Here's how the part is built. I have some questions about the finished solid (model axes, mm). A direction names the side the tool comes from. Coordinates: 2 decimals unless noted, no trailing zeros. Order: outer loops, then holes, each group sorted by start corner. A loop starts at its lowest first (then second) coordinate and runs counter-clockwise, first axis right, second up. Notation, with made-up numbers: (53, 87.5) - (91, 87.5) arc R8 cw to (91, 97.5) - close; hole circle Ø1 at (-25.5, -36). An arc over 180 degrees is marked (long way). Answer in a Markdown table with one row per item. Add a question column.
Item 1: Will these pins go through, and if not, where does the flat tip stop? pin 1 Ø4 at (x, z) = (85, 4) entering from -Y; pin 2 Ø1.5 at (x, z) = (6.5, 4) entering from -Y; pin 3 Ø3.5 at (y, z) = (44.5, 3) entering from -X; pin 4 Ø2.5 at (y, z) = (72.5, 4) entering from -X.
Item 2: I want a section at C-C (y = 18). Please give me the cut outline in (x, z).
Item 3: I want a section at D-D (x = 6). Please give me the cut outline in (y, z), plus the area to 3 significant figures.
Item 4: I want a section at B-B (z = 4). Count the separate pieces of the cut face and the enclosed holes in it, plus the area to 3 significant figures.
Item 5: If I drill on line 1 along Z through (x, y) = (6, 11); line 2 along X through (y, z) = (13.5, 3.5); line 3 along Y through (x, z) = (90, 6.75), over which ranges is the centre line in solid material (lowest first)? Write a range as from..to.
Item 6: I want a section at A-A (x = 20). Please give me the cut outline in (y, z), plus the area to 4 significant figures.
Item 7: On a 3-axis mill with a long thin cutter (end or side, diameter ignored), from which of +Z, -Z, +X, -X, +Y, -Y can I reach the whole of each face in a straight line? I mean faces 5 (the flat face through (85, 45, 4)), 6 (the flat face through (26, 52, 4)), 7 (the cylindrical face through (80.942, 14.35, 2.465)), 8 (the cylindrical face through (56, 37.8, 3.9)). Say none if no direction works.
Item 8: Thinking about a two-plate mould opening in X: for faces 1 (the cylindrical face through (56, 49.2, 3.9)), 2 (the flat face through (46, 0, 4)), 3 (the flat face through (88, 20, 4)), 4 (the cylindrical face through (4.51, 47.72, 4.06)), which applies, +X half, -X half, draft (parallel to the pull), parting line (faces both ways), or undercut?
```python
from build123d import *

# Parameters (mm, degrees)
BOSS_EXTRU_1_DEPTH      = 8
ESQUISSE2_R             = 7.95
ENL_V_MAT_EXTRU_1_DEPTH = 5
ESQUISSE3_R             = 6
ENL_V_MAT_EXTRU_2_DEPTH = 4
ENL_V_MAT_EXTRU_3_DEPTH = 9
ESQUISSE5_R             = 1.5
ENL_V_MAT_EXTRU_4_DEPTH = 30
CONG_1_R                = 15
ESQUISSE6_R             = 1.5
ENL_V_MAT_EXTRU_5_DEPTH = 20


with BuildPart() as part:
    # Esquisse1 → Boss.-Extru.1 (new body)
    with BuildSketch(Plane.XY):
        Polygon((52, 75), (52, 52), (0, 52), (0, 0), (94, 0), (94, 75), align=None)
    extrude(amount=BOSS_EXTRU_1_DEPTH)

    # Esquisse2 → Enlèv. mat.-Extru.1 (cut)
    with BuildSketch(Plane(origin=(0, 0, 0), x_dir=(-1, 0, 0), z_dir=(0, 0, -1))):
        with Locations((-20, 18)):
            Circle(ESQUISSE2_R)
        with Locations((-73, 14)):
            Circle(ESQUISSE2_R)
    extrude(amount=-ENL_V_MAT_EXTRU_1_DEPTH, mode=Mode.SUBTRACT)

    # Esquisse3 → Enlèv. mat.-Extru.2 (cut, through all)
    with BuildSketch(Plane(origin=(0, 0, 5), x_dir=(-1, 0, 0), z_dir=(0, 0, -1))):
        with Locations((-73, 14)):
            Circle(ESQUISSE3_R)
        with Locations((-20, 18)):
            Circle(ESQUISSE3_R)
    extrude(amount=-ENL_V_MAT_EXTRU_2_DEPTH, mode=Mode.SUBTRACT)

    # Esquisse4 → Enlèv. mat.-Extru.3 (cut, through all)
    with BuildSketch(Plane(origin=(0, 0, 0), x_dir=(-1, 0, 0), z_dir=(0, 0, -1))):
        with BuildLine():
            Line((-92.2, 40), (-92.2, 47))
            ThreePointArc((-92.2, 47), (-90, 49.2), (-87.8, 47))
            Line((-87.8, 47), (-87.8, 40))
            ThreePointArc((-87.8, 40), (-90, 37.8), (-92.2, 40))
        make_face()
        with BuildLine():
            Line((-53.8, 40), (-53.8, 47))
            ThreePointArc((-53.8, 47), (-56, 49.2), (-58.2, 47))
            Line((-58.2, 47), (-58.2, 40))
            ThreePointArc((-58.2, 40), (-56, 37.8), (-53.8, 40))
        make_face()
    extrude(amount=-ENL_V_MAT_EXTRU_3_DEPTH, mode=Mode.SUBTRACT)

    # Esquisse5 → Enlèv. mat.-Extru.4 (cut)
    with BuildSketch(Plane(origin=(0, 75, 0), x_dir=(1, 0, 0), z_dir=(0, 1, 0))):
        with Locations((61, -4)):
            Circle(ESQUISSE5_R)
        with Locations((85, -4)):
            Circle(ESQUISSE5_R)
    extrude(amount=-ENL_V_MAT_EXTRU_4_DEPTH, mode=Mode.SUBTRACT)

    # Congé1
    cong_1_edges = [part.edges().sort_by_distance(p)[0] for p in [
        (0, 52, 4),
        (52, 52, 4),
    ]]
    fillet(cong_1_edges, radius=CONG_1_R)

    # Esquisse6 → Enlèv. mat.-Extru.5 (cut)
    with BuildSketch(Plane.XZ):
        with Locations((6, 4)):
            Circle(ESQUISSE6_R)
        with Locations((88, 4)):
            Circle(ESQUISSE6_R)
    extrude(amount=-ENL_V_MAT_EXTRU_5_DEPTH, mode=Mode.SUBTRACT)


solid = part.part
```
Values follow:
| question | item | result |
|---|---|---|
| 1 | pin 1 | stops at y = 0 |
| 1 | pin 2 | stops at y = 20 |
| 1 | pin 3 | stops at x = 1.15 |
| 1 | pin 4 | stops at x = 52 |
| 2 | outline | (0, 0) - (12.05, 0) - (12.05, 5) - (14, 5) - (14, 8) - (0, 8) - close; (26, 5) - (27.95, 5) - (27.95, 0) - (66.13, 0) - (66.13, 5) - (68.53, 5) - (68.53, 8) - (26, 8) - close; (77.47, 5) - (79.87, 5) - (79.87, 0) - (94, 0) - (94, 8) - (77.47, 8) - close; hole circle Ø3 at (6, 4); hole circle Ø3 at (88, 4) |
| 3 | outline | (0, 0) - (49, 0) - (49, 8) - (0, 8) - (0, 5.5) - (20, 5.5) - (20, 2.5) - (0, 2.5) - close |
| 3 | area | 332 mm^2 |
| 4 | separate pieces | 1 |
| 4 | enclosed holes | 4 |
| 4 | area | 5,060 mm^2 |
| 5 | line 1 | z = 0..2.5, 5.5..8 |
| 5 | line 2 | x = 0..4.59, 7.41..13.45, 26.55..65.07, 80.93..86.59, 89.41..94 |
| 5 | line 3 | y = 0..37.8, 49.2..75 |
| 6 | outline | (0, 0) - (10.05, 0) - (10.05, 5) - (12, 5) - (12, 8) - (0, 8) - close; (24, 5) - (25.95, 5) - (25.95, 0) - (52, 0) - (52, 8) - (24, 8) - close |
| 6 | area | 300.5 mm^2 |
| 7 | face 5 | +Y |
| 7 | face 6 | +Z, -Z, -X, +Y |
| 7 | face 7 | -Z |
| 7 | face 8 | +Z, -Z |
| 8 | face 1 | undercut |
| 8 | face 2 | draft |
| 8 | face 3 | undercut |
| 8 | face 4 | -X half |
